Autodesk Inventor part; units mm, degrees
ref_plane "metal_to_body_XY" through (-0.508, 0, 0) normal (1, 0, 0) x (0, 0, -1)
ref_plane "metal_to_body_YZ" through (-0.508, 0, 0) normal (0, 0, -1) x (0, 1, 0)
ref_plane "metal_to_body_ZX" through (-0.508, 0, 0) normal (0, 1, 0) x (1, 0, 0)
sketch "Sketch_1" plane through (0, 0, 7.9756) normal (0, 0, 1) x (1, 0, 0)
  line L0 (-8.2677, 3.0734) -> (-4.8133, 3.0734)
  line L1 (-4.8133, 3.0734) -> (-4.8133, 8.1534)
  line L2 (-4.8133, 8.1534) -> (-8.2677, 8.1534)
  line L3 (-8.2677, 8.1534) -> (-8.2677, 3.0734)
  line L4 (-7.0993, 6.2484) -> (-7.0993, 4.6228)
  line L5 (-7.0993, 4.6228) -> (-5.9817, 4.6228)
  line L6 (-5.9817, 4.6228) -> (-5.9817, 6.2484)
  line L7 (-5.9817, 6.2484) -> (-7.0993, 6.2484)
extrude "Extrusion1" add sketch "Sketch_1" against normal blind 0.254
sketch "Sketch_2" plane through (0, 7.9502, 0) normal (0, 1, 0) x (1, 0, 0)
  line L0 (-7.0993, 7.9756) -> (-7.0993, -7.9756)
  line L1 (-7.0993, -7.9756) -> (-4.8133, -7.9756)
  line L2 (-4.8133, -7.9756) -> (-4.8133, 7.9756)
  line L3 (-4.8133, 7.9756) -> (-7.0993, 7.9756)
extrude "Extrusion2" add sketch "Sketch_2" along normal blind 0.2032
sketch "Sketch_3" plane through (0, 0, -7.9756) normal (0, 0, 1) x (1, 0, 0)
  line L0 (-8.2677, 3.0734) -> (-4.8133, 3.0734)
  line L1 (-4.8133, 3.0734) -> (-4.8133, 8.1534)
  line L2 (-4.8133, 8.1534) -> (-8.2677, 8.1534)
  line L3 (-8.2677, 8.1534) -> (-8.2677, 3.0734)
  line L4 (-7.0993, 6.2484) -> (-7.0993, 4.6228)
  line L5 (-7.0993, 4.6228) -> (-5.9817, 4.6228)
  line L6 (-5.9817, 4.6228) -> (-5.9817, 6.2484)
  line L7 (-5.9817, 6.2484) -> (-7.0993, 6.2484)
extrude "Extrusion3" add sketch "Sketch_3" along normal blind 0.254
sketch "Sketch_5" plane through (0, 0, 0) normal (0, 0, 1) x (1, 0, 0)
  line L0 (-12.0887, 8.8412) -> (-7.0358, 7.9502)
  line L1 (-7.0358, 7.9502) -> (-7.0005, 8.1503)
  line L2 (-7.0005, 8.1503) -> (-12.0534, 9.0413)
  line L3 (-12.0534, 9.0413) -> (-12.0887, 8.8412)
extrude "Extrusion4" add sketch "Sketch_5" along normal mid plane 15.4432
sketch "Sketch_6" plane through (0, 7.9502, 0) normal (0, 1, 0) x (1, 0, 0)
  line L0 (-15.494, -7.7216) -> (-6.985, -7.7216)
  line L1 (-6.985, -7.7216) -> (-6.985, -7.0866)
  line L2 (-6.985, -7.0866) -> (-14.732, -7.0866)
  line L3 (-14.732, -7.0866) -> (-14.732, -6.1666)
  line L4 (-14.732, -6.1666) -> (-6.985, -4.8006)
  line L5 (-6.985, -4.8006) -> (-6.985, 4.8006)
  line L6 (-6.985, 4.8006) -> (-14.732, 6.1666)
  line L7 (-14.732, 6.1666) -> (-14.732, 7.0866)
  line L8 (-14.732, 7.0866) -> (-6.985, 7.0866)
  line L9 (-6.985, 7.0866) -> (-6.985, 7.7216)
  line L10 (-6.985, 7.7216) -> (-15.494, 7.7216)
  line L11 (-15.494, 7.7216) -> (-15.494, -7.7216)
extrude "Extrusion5" cut sketch "Sketch_6" along normal blind 2.54
ref_plane "metal_to_body_XY" through (-0.508, 0, 0) normal (1, 0, 0) x (0, 0, -1)
ref_plane "metal_to_body_YZ" through (-0.508, 0, 0) normal (0, 0, -1) x (0, 1, 0)
ref_plane "metal_to_body_ZX" through (-0.508, 0, 0) normal (0, 1, 0) x (1, 0, 0)
properties part number "UB216KKW015C-NR"
Check sheet for the modelled part. Datum: model origin and axes. Units: mm. A direction names the side the tool comes from. Round coordinates to 2 decimals unless told otherwise and drop trailing zeros. Loops run counter-clockwise (first coordinate to the right, second up) from the corner with the lowest first, then second, coordinate; pieces in that order, holes last.
1. Sectioned sample at D-D on x = -8. Record the boundary of the cut face in (y, z), and give its area (3 significant figures).
2. Sectioned sample at B-B on x = -6.25. Record the boundary of the cut face in (y, z), and give its area (3 significant figures).
3. Sectioned sample at C-C on x = -9.25. Record the boundary of the cut face in (y, z), and give its area (3 significant figures).
4. Gauge pin test, flat ends, axial feed: pin 1 Ø1.1 at (x, z) = (-6, 1) entering from -Y; pin 2 Ø1 at (y, z) = (8.5, -4) entering from -X (3 decimals); pin 3 Ø0.9 at (x, y) = (-10.5, 8.5) entering from +Z. Record the tip position at first contact, or that the pin passes through.
5. Set-up check for faces 4 (the flat face through (-6, 7.95, 0)), 5 (the flat face through (-9.5, 8.59, -6.22)), 6 (the flat face through (-9.629, 8.407, -6.221)): record each of +Z, -Z, +X, -X, +Y, -Y from which the full face is reachable in a straight line by a thin tool's end or side.
6. Mould release check, pull along Z, two halves, no side actions. Record for faces 1 (the flat face through (-7.3, 5.6, 7.976)), 2 (the flat face through (-7.3, 5.6, 7.722)), 3 (the flat face through (-9.5, 8.59, 6.18)): released by +Z, released by -Z, zero draft, split by the parting line, or undercut.
7. Sectioned sample at A-A on y = 6.8. Record the boundary of the cut face in (x, z).
8. Scan lines: probe 1 along Z at (x, y) = (-7, 7.85); probe 2 along Y at (x, z) = (-6.25, 3.25); probe 3 along Z at (x, y) = (-11, 8.75). Record each from-to range of solid material in increasing order.
Recorded:
1. outline: (3.07, -7.98) - (8.15, -7.98) - (8.15, -7.72) - (3.07, -7.72) - close; (3.07, 7.72) - (8.15, 7.72) - (8.15, 7.98) - (3.07, 7.98) - close; (8.12, -7.09) - (8.33, -7.09) - (8.33, -4.98) - (8.12, -4.98) - close; (8.12, 4.98) - (8.33, 4.98) - (8.33, 7.09) - (8.12, 7.09) - close
1. area: 3.45 mm2
2. outline: (3.07, -7.98) - (4.62, -7.98) - (4.62, -7.72) - (3.07, -7.72) - close; (3.07, 7.72) - (4.62, 7.72) - (4.62, 7.98) - (3.07, 7.98) - close; (6.25, -7.98) - (8.15, -7.98) - (8.15, 7.98) - (6.25, 7.98) - (6.25, 7.72) - (7.95, 7.72) - (7.95, -7.72) - (6.25, -7.72) - close
2. area: 4.89 mm2
3. outline: (8.34, -7.09) - (8.55, -7.09) - (8.55, -5.2) - (8.34, -5.2) - close; (8.34, 5.2) - (8.55, 5.2) - (8.55, 7.09) - (8.34, 7.09) - close
3. area: 0.779 mm2
4. pin 1: stops at y = 7.95
4. pin 2: stops at x = -6.985
4. pin 3: stops at z = 7.09
5. face 4: +X, -X, -Y
5. face 5: +Z, -Z, +X, +Y
5. face 6: -X, -Y
6. face 1: released by +Z
6. face 2: undercut
6. face 3: zero draft
7. outline: (-8.27, -7.98) - (-4.81, -7.98) - (-4.81, -7.72) - (-8.27, -7.72) - close; (-8.27, 7.72) - (-4.81, 7.72) - (-4.81, 7.98) - (-8.27, 7.98) - close
8. probe 1: z = -7.98 to -7.72, 7.72 to 7.98
8. probe 2: y = 7.95 to 8.15
8. probe 3: z = -7.09 to -5.51, 5.51 to 7.09
